Source: CAD feature listing. Evaluate the final solid. Frame: model axes, mm. Coordinates: 2 decimals unless noted, no trailing zeros. Order: outer loops, then holes, each group sorted by start corner. A loop starts at its lowest first (then second) coordinate and runs counter-clockwise, first axis right, second up.
```python
from build123d import *

# Parameters (mm, degrees)
IZIM1_W                     = 60
IZIM1_H                     = 60
IZIM1_R                     = 18.5
IZIM1_R_2                   = 6
Y_KSEKLIK_EKSTR_ZYON1_DEPTH = 10


with BuildPart() as part:
    # Çizim1 → Yükseklik-Ekstrüzyon1 (new body)
    with BuildSketch(Plane.XY):
        Rectangle(IZIM1_W, IZIM1_H)
        Circle(IZIM1_R, mode=Mode.SUBTRACT)
        with Locations((20, 20)):
            Circle(IZIM1_R_2, mode=Mode.SUBTRACT)
        with Locations((-20, 20)):
            Circle(IZIM1_R_2, mode=Mode.SUBTRACT)
        with Locations((20, -20)):
            Circle(IZIM1_R_2, mode=Mode.SUBTRACT)
        with Locations((-20, -20)):
            Circle(IZIM1_R_2, mode=Mode.SUBTRACT)
    extrude(amount=Y_KSEKLIK_EKSTR_ZYON1_DEPTH)


solid = part.part
```
1. Section query A-A on x = 0. Return loops of the section in (y, z), plus the area to 3 significant figures.
Findings:
outline: (-30, 0) - (-18.5, 0) - (-18.5, 10) - (-30, 10) - close; (18.5, 0) - (30, 0) - (30, 10) - (18.5, 10) - close
area: 230 mm2
2. Section query B-B on z = 3. Return loops of the section in (x, y), plus the area to 3 significant figures.
Findings:
outline: (-30, -30) - (30, -30) - (30, 30) - (-30, 30) - close; hole circle Ø12 at (-20, -20); hole circle Ø12 at (-20, 20); hole circle Ø37 at (0, 0); hole circle Ø12 at (20, -20); hole circle Ø12 at (20, 20)
area: 2,070 mm2
3. Ray query, line 1 (Y direction, x = -20, z = 5.75); line 2 (X direction, y = 17, z = 6.5); line 3 (Y direction, x = 25.5, z = 8.5). Return the intervals inside material, ascending.
Findings:
line 1: y = -30 to -26, -14 to 14, 26 to 30
line 2: x = -30 to -25.2, -14.8 to -7.3, 7.3 to 14.8, 25.2 to 30
line 3: y = -30 to -22.4, -17.6 to 17.6, 22.4 to 30
4. Draft query along Y for faces 1 (the face through (30, 0, 5)), 2 (the face through (-24.76, 16.35, 4.93)), 3 (the face through (0, 30, 5)), 4 (the face through (0, -30, 5)). Return one class per face: released by +Y, released by -Y, zero draft, split by the parting line, or undercut.
Findings:
face 1: zero draft
face 2: undercut
face 3: released by +Y
face 4: released by -Y
5. Section query D-D on y = 20. Return loops of the section in (x, z), plus the area to 3 significant figures.
Findings:
outline: (-30, 0) - (-26, 0) - (-26, 10) - (-30, 10) - close; (-14, 0) - (14, 0) - (14, 10) - (-14, 10) - close; (26, 0) - (30, 0) - (30, 10) - (26, 10) - close
area: 360 mm2
